The listing builds one solid part. Answer for the finished solid, in the listing's coordinates (mm). A direction names the side the tool comes from. Give positions to 0.01 mm unless a question says otherwise; leave off trailing zeros. Loops run counter-clockwise (first coordinate to the right, second up) from the corner with the lowest first, then second, coordinate; pieces in that order, holes last.
Item 1: Section B-B, the plane z = -12 is taken. Give the vertices of the cut face in (x, y).
Item 2: Section C-C, the plane x = 16 is taken. Give the vertices of the cut face in (y, z), and give its area (3 significant figures).
Item 3: Section D-D, the plane y = 58.5 is taken. Give the vertices of the cut face in (x, z), and give its area (3 significant figures).
Item 4: Section A-A, the plane z = -1 is taken. Give the vertices of the cut face in (x, y), and give its area (3 significant figures).
Item 5: Each of these flat-tipped pins is pushed along its axis until it touches: pin 1 Ø4 at (y, z) = (65.5, 3.5) entering from -X; pin 2 Ø14.5 at (x, z) = (28, -14) entering from -Y; pin 3 Ø1.2 at (x, y) = (27.5, 33.1) entering from +Z; pin 4 Ø17.5 at (x, z) = (28, 20) entering from +Y. Where does it stop, or does it pass through?
Item 6: Consider line 1 along Y through (x, z) = (27.5, 3.75); line 2 along Y through (x, z) = (16, -14.5); line 3 along X through (y, z) = (54.5, -6). Determine where each line is inside the solid, lowest interval first.
Item 7: The mould has two halves that part along Z. Classify faces 4 (the face through (7.04, 26.53, 15.85)), 5 (the face through (39, 65, -5)), 6 (the face through (22.5, 27, -5)), 7 (the face through (10, 65, 17)): pulls with the +Z half, pulls with the -Z half, needs draft (parallel to the pull), parting line crosses it, or undercut.
Item 8: A tool of negligible diameter and unlimited length cuts with its end or side. For faces 1 (the face through (25, 5, 19)), 2 (the face through (36.5, 46, -10)), 3 (the face through (38.5, 65.07, 22.07)), from which of +Z, -Z, +X, -X, +Y, -Y can it reach the whole face along a straight path? Write none if from no direction.
Autodesk Inventor part; units mm, degrees
ref_plane "YZ Plane" through (0, 0, 0) normal (1, 0, 0) x (0, 1, 0)
ref_plane "XZ Plane" through (0, 0, 0) normal (0, 1, 0) x (-1, 0, 0)
ref_plane "XY Plane" through (0, 0, 0) normal (0, 0, 1) x (1, 0, 0)
sketch "Sketch1" plane through (0, 0, 0) normal (0, 0, 1) x (1, 0, 0)
  line L0 (0, 0) -> (50, 0)
  line L1 (50, 0) -> (50, 75)
  line L2 (50, 75) -> (0, 75)
  line L3 (0, 75) -> (0, 0)
  dimension "d0" = 50
  dimension "d1" = 75
extrude "Extrusion1" add sketch "Sketch1" along normal blind 5
sketch "Sketch2" plane through (0, 0, 0) normal (0, 1, 0) x (-1, 0, 0)
  line L0 (0, 5) -> (-50, 5)
  line L1 (0, 5) -> (-50, 5)
  line L2 (-50, 5) -> (-50, 27)
  line L3 (-50, 27) -> (0, 27)
  line L4 (0, 27) -> (0, 5)
  point P0 (0, 0)
  dimension "d4" = 22
extrude "Extrusion2" add sketch "Sketch2" along normal blind 5
sketch "Sketch3" plane through (0, 0, 5) normal (0, 0, 1) x (1, 0, 0)
  circle A0 centre (42.5, 30) radius 3.5
  circle A1 centre (40, 65) radius 3.5
  circle A2 centre (10, 65) radius 3.5
  circle A3 centre (7.5, 30) radius 3.5
  line L0 (42.5, 30) -> (7.5, 30) construction
  line L1 (50, 75) -> (0, 75) construction
  line L2 (25, 75) -> (25, 30) construction
  line L3 (10, 65) -> (40, 65) construction
  point P0 (0, 0)
  point P1 (25, 65)
  dimension "d7" = 7
  dimension "d8" = 7
  dimension "d9" = 7
  dimension "d10" = 7
  dimension "d12" = 30
  dimension "d14" = 10
  dimension "d30" = 35
  dimension "d32" = 35
extrude "Extrusion3" add sketch "Sketch3" along normal blind 22
sketch "Sketch4" plane through (40, 65, 27) normal (0, 0, 1) x (1, 0, 0)
  circle A0 centre (-30, 0) radius 3.5
  circle A1 centre (0, 0) radius 3.5
  circle A2 centre (2.5, -35) radius 3.5
  circle A3 centre (-32.5, -35) radius 3.5
  circle A4 centre (-30, 0) radius 1.5
  circle A5 centre (0, 0) radius 1.5
  circle A6 centre (2.5, -35) radius 1.5
  circle A7 centre (-32.5, -35) radius 1.5
  point P0 (-40, -65)
  dimension "d17" = 3
  dimension "d18" = 3
  dimension "d19" = 3
  dimension "d20" = 3
extrude "Extrusion4" cut sketch "Sketch4" against normal blind 10 contours A4 | A5 | A6 | A7
sketch "Sketch5" plane through (0, 5, 0) normal (0, 1, 0) x (1, 0, 0)
  circle A0 centre (25, -16) radius 2.5
  line L0 (0, -5) -> (50, -5)
  line L1 (0, -5) -> (0, -27)
  line L2 (0, -27) -> (50, -27)
  line L3 (50, -27) -> (50, -5)
  point P0 (0, 0)
  point P1 (0, -16)
  point P2 (25, -27)
  dimension "d23" = 5
extrude "Extrusion5" cut sketch "Sketch5" against normal through all contours A0
sketch "Sketch6" plane through (0, 0, 5) normal (0, 0, 1) x (1, 0, 0)
  circle A0 centre (10, 65) radius 3.5
  circle A1 centre (40, 65) radius 3.5
  circle A2 centre (10, 65) radius 1.5
  circle A3 centre (10, 65) radius 7.5
  circle A4 centre (40, 65) radius 7.5
  point P0 (0, 0)
  dimension "d26" = 15
  dimension "d27" = 15
extrude "Extrusion6" add sketch "Sketch6" along normal blind 10 contours A3 | A4
sketch "Sketch8" plane through (0, 0, 0) normal (0, 0, -1) x (-1, 0, 0)
  circle A0 centre (-42.5, 30) radius 1.5
  circle A1 centre (-42.5, 30) radius 20
  circle A2 centre (-7.5, 30) radius 3.5
  circle A3 centre (-7.5, 30) radius 20
  point P0 (0, 0)
  dimension "d33" = 40
  dimension "d34" = 40
extrude "Extrusion7" add sketch "Sketch8" against normal blind 5 contours A1 A3 | A1 A3 | A3 A1 | A2
sketch "Sketch9" plane through (0, 0, 5) normal (0, 0, 1) x (1, 0, 0)
  circle A0 centre (27.5, 50.5) radius 5.5
  line L0 (50, 75) -> (0, 75)
  line L1 (50, 75) -> (0, 75) construction
  line L2 (25, 75) -> (25, 35.564) construction
  point P0 (0, 0)
  dimension "d37" = 11
  dimension "d38" = 24.5
  dimension "d39" = 2.5
extrude "Extrusion8" cut sketch "Sketch9" against normal through all
sketch "Sketch10" plane through (0, 0, 5) normal (0, 0, 1) x (1, 0, 0)
  circle A0 centre (27.5, 58.5) radius 1
  circle A1 centre (27.5, 33.1) radius 1
  line L0 (27.5, 58.5) -> (27.5, 33.1) construction
  circle A2 centre (27.5, 50.5) radius 5.5
  point P0 (0, 0)
  dimension "d42" = 2
  dimension "d43" = 2
  dimension "d44" = 25.4
  dimension "d45" = 8
extrude "Extrusion9" cut sketch "Sketch10" against normal through all contours A0 | A1
sketch "Sketch11" plane through (0, 0, 0) normal (0, 0, -1) x (-1, 0, 0)
  circle A0 centre (-27.5, 58.5) radius 1
  circle A1 centre (-27.5, 33.1) radius 1
  circle A2 centre (-27.5, 58.5) radius 2.5
  circle A3 centre (-27.5, 33.1) radius 2.5
  point P0 (0, 0)
  dimension "d48" = 1.5
  dimension "d49" = 1.5
extrude "Extrusion10" add sketch "Sketch11" along normal blind 4
sketch "Sketch12" plane through (0, 0, 0) normal (0, 0, -1) x (-1, 0, 0)
  line L0 (-36.5, 29.1) -> (-18.5, 29.1)
  line L1 (-18.5, 29.1) -> (-18.5, 62.5)
  line L2 (-18.5, 62.5) -> (-36.5, 62.5)
  line L3 (-36.5, 62.5) -> (-36.5, 29.1)
  circle A0 centre (-27.5, 50.5) radius 5.5
  line L4 (-50, 75) -> (0, 75)
  line L5 (-41.5, 24.1) -> (-13.5, 24.1)
  line L6 (-13.5, 24.1) -> (-13.5, 67.5)
  line L7 (-13.5, 67.5) -> (-41.5, 67.5)
  line L8 (-41.5, 67.5) -> (-41.5, 24.1)
  circle A1 centre (-27.5, 58.5) radius 1
  circle A2 centre (-27.5, 33.1) radius 1
  point P0 (0, 0)
  point P1 (-26.1358, 55.8281)
  point P2 (-28.8642, 55.8281)
  point P3 (-27.5, 62.5)
  dimension "d52" = 18
  dimension "d55" = 5
  dimension "d58" = 4
  dimension "d59" = 4
extrude "Extrusion11" add sketch "Sketch12" along normal blind 20 contours L8 L7 L6 L5
sketch "Sketch13" plane through (0, 0, -20) normal (0, 0, -1) x (-1, 0, 0)
  line L0 (-36.5, 29.1) -> (-36.5, 62.5) construction
  line L1 (-36.5, 62.5) -> (-18.5, 62.5) construction
  line L2 (-18.5, 62.5) -> (-18.5, 29.1) construction
  line L3 (-18.5, 29.1) -> (-36.5, 29.1) construction
  line L4 (-41.5, 24.1) -> (-13.5, 24.1) construction
  line L5 (-13.5, 24.1) -> (-13.5, 67.5) construction
  line L6 (-13.5, 67.5) -> (-41.5, 67.5) construction
  line L7 (-41.5, 67.5) -> (-41.5, 24.1) construction
  line L8 (-39, 65) -> (-16, 65) construction
  line L9 (-16, 65) -> (-16, 26.6) construction
  line L10 (-16, 26.6) -> (-39, 26.6) construction
  line L11 (-39, 26.6) -> (-39, 65) construction
  circle A0 centre (-39, 65) radius 1.5
  circle A1 centre (-16, 65) radius 1.5
  circle A2 centre (-16, 26.6) radius 1.5
  circle A3 centre (-39, 26.6) radius 1.5
  point P0 (0, 0)
  dimension "d60" = 2.5
  dimension "d61" = 3
  dimension "d62" = 3
  dimension "d63" = 3
  dimension "d64" = 3
extrude "Extrusion12" cut sketch "Sketch13" against normal blind 15
sketch "Sketch14" plane through (13.5, 24.1, 0) normal (0, -1, 0) x (1, 0, 0)
  line L0 (28, 0) -> (0, 0)
  line L1 (19, 0) -> (9, 0)
  line L2 (9, 0) -> (9, -10)
  line L3 (9, -10) -> (19, -10)
  line L4 (19, -10) -> (19, 0)
  line L5 (0, 0) -> (28, 0)
  point P0 (-13.5, 0)
  point P1 (14, 0)
  dimension "d67" = 10
  dimension "d68" = 10
extrude "Extrusion13" cut sketch "Sketch14" against normal blind 5
sketch "Sketch15" plane through (0, 0, 0) normal (0, 0, -1) x (-1, 0, 0)
  circle A0 centre (-27.5, 50.5) radius 5.5
  circle A1 centre (-27.5, 45) radius 4
  point P0 (0, 0)
  dimension "d71" = 8
extrude "Extrusion14" cut sketch "Sketch15" against normal through all contours A1 A0 | A0 A1 picked at (-26.7332, 46.3513) picked at (-26.5311, 43.8278)
equation "\"d49\" = d48"
properties part number "GA001" material "ABS Plastic"
Worked answers:
1. outline: (13.5, 24.1) - (41.5, 24.1) - (41.5, 67.5) - (13.5, 67.5) - close; hole circle Ø3 at (16, 26.6); hole circle Ø3 at (16, 65); hole (18.5, 29.1) - (36.5, 29.1) - (36.5, 62.5) - (18.5, 62.5) - close; hole circle Ø3 at (39, 26.6); hole circle Ø3 at (39, 65)
2. outline: (0, 0) - (24.1, 0) - (24.1, -20) - (25.1, -20) - (25.1, -5) - (28.1, -5) - (28.1, -20) - (63.5, -20) - (63.5, -5) - (66.5, -5) - (66.5, -20) - (67.5, -20) - (67.5, 0) - (75, 0) - (75, 5) - (69.5, 5) - (69.5, 15) - (60.5, 15) - (60.5, 5) - (5, 5) - (5, 27) - (0, 27) - close
2. area: 1,350 mm2
3. outline: (0, 0) - (13.5, 0) - (13.5, -20) - (18.5, -20) - (18.5, 0) - (25, 0) - (25, -4) - (26.5, -4) - (26.5, 5) - (13.74, 5) - (13.74, 15) - (6.26, 15) - (6.26, 5) - (0, 5) - close; (28.5, -4) - (30, -4) - (30, 0) - (36.5, 0) - (36.5, -20) - (41.5, -20) - (41.5, 0) - (50, 0) - (50, 5) - (43.74, 5) - (43.74, 15) - (36.26, 15) - (36.26, 5) - (28.5, 5) - close
3. area: 602 mm2
4. outline: (13.5, 24.1) - (22.5, 24.1) - (22.5, 29.1) - (18.5, 29.1) - (18.5, 62.5) - (36.5, 62.5) - (36.5, 29.1) - (32.5, 29.1) - (32.5, 24.1) - (41.5, 24.1) - (41.5, 67.5) - (13.5, 67.5) - close; circle Ø5 at (27.5, 33.1); circle Ø5 at (27.5, 58.5); hole circle Ø2 at (27.5, 33.1); hole circle Ø2 at (27.5, 58.5)
4. area: 597 mm2
5. pin 1: stops at x = 0
5. pin 2: stops at y = 24.1
5. pin 3: passes through
5. pin 4: stops at y = 70.75
6. line 1: y = 0 to 32.1, 34.1 to 41, 56 to 57.5, 59.5 to 75
6. line 2: y = 24.1 to 25.1, 28.1 to 63.5, 66.5 to 67.5
6. line 3: x = 13.5 to 18.5, 36.5 to 41.5
7. face 4: needs draft
7. face 5: pulls with the -Z half
7. face 6: undercut
7. face 7: pulls with the +Z half
8. face 1: +Z, +X, -X
8. face 2: -Z
8. face 3: +Z
